The model under review builds one solid part; all positions refer to its coordinate system, in mm. A direction names the side the tool comes from. Round coordinates to 2 decimals unless told otherwise and drop trailing zeros. Write each loop counter-clockwise with the first axis right and the second up, starting at its lowest first coordinate (ties: lowest second). Pieces come first, ordered by that corner, then holes.
Item 1: To check wall thickness, follow L1, parallel to Z at x = 3, y = 260; L2, parallel to Y at x = 27, z = 490; L3, parallel to X at y = 1, z = 622. State the ranges of each line that lie inside material, in increasing order.
Item 2: Draft analysis for pull direction Y (two halves, no side actions). For faces 1 (the face through (4, 270, 0)), 2 (the face through (39, 0, 715)), 3 (the face through (2.465, 155.66, 379.993)), state which applies: +Y half, -Y half, draft (parallel to the pull), parting line (faces both ways), or undercut.
Item 3: Clearance check with flat-ended pins moving along their axes: pin 1 Ø22 at (y, z) = (280, 375) entering from +X; pin 2 Ø5.5 at (x, z) = (1.5, 257.5) entering from -Y; pin 3 Ø9 at (x, z) = (40.09, 640) entering from -Y. State where each tip first meets the part, or that it passes through.
Item 4: Machinability: for faces 4 (the face through (39, 310, 715)), 5 (the face through (5, 157, 715)), which of the approach directions +Z, -Z, +X, -X, +Y, -Y give a long, thin tool a straight path to every point of the face, cutting with its end or side? Answer none if there is none.
Item 5: Add section A-A (z = 1319). Give the boundary of the cut face in (x, y), plus the area to 3 significant figures.
```python
from build123d import *

# Parameters (mm, degrees)
EXTRUDE_1_DEPTH             = 1450
CUT_EXTRUDE_705_DEPTH       = 10
SKETCH_3_R                  = 8.5
CUT_EXTRUDE_1476_DEPTH      = 5
SKETCH_9_R                  = 4
CUT_EXTRUDE_2268_DEPTH      = 10
SKETCH_12_R                 = 6.6
CUT_EXTRUDE_3079_DEPTH      = 10
CUT_EXTRUDE_3564_DEPTH      = 10
SKETCH_17_R                 = 6.6
CUT_EXTRUDE_3911_DEPTH      = 10
FILLET_1_R                  = 10
SKETCH_21_R                 = 4.1
CUT_EXTRUDE_1_DEPTH         = 5
SKETCH_22_R                 = 5.5
CUT_EXTRUDE_4798_DEPTH      = 5
SKETCH_23_R                 = 8.25
CUT_EXTRUDE_5030_DEPTH      = 10
SKETCH_24_R                 = 4.1
CUT_EXTRUDE_2_DEPTH         = 10
HOLE_WIZARD_M61_D           = 6.6
HOLE_WIZARD_M61_DEPTH       = 10
HOLE_WIZARD_M61_CSINK_D     = 13.71
HOLE_WIZARD_M61_CSINK_ANGLE = 90
HOLE_WIZARD_M61_TIP         = 1.982840043


with BuildPart() as part:
    # Эскиз1 → Бобышка-Вытянуть1 (new body)
    with BuildSketch(Plane.XY):
        with BuildLine():
            Line((70, 0), (8, 0))
            ThreePointArc((8, 0), (2.343145751, 2.343145751), (0, 8))
            Line((0, 8), (0, 302))
            ThreePointArc((0, 302), (2.343145751, 307.656854249), (8, 310))
            Line((8, 310), (70, 310))
            Line((70, 310), (70, 305))
            Line((70, 305), (8, 305))
            ThreePointArc((8, 305), (5.878679656, 304.121320344), (5, 302))
            Line((5, 302), (5, 8))
            ThreePointArc((5, 8), (5.878679656, 5.878679656), (8, 5))
            Line((8, 5), (70, 5))
            Line((70, 5), (70, 0))
        make_face()
    extrude(amount=EXTRUDE_1_DEPTH)

    # Эскиз2 → Cut-Extrude 705 (cut)
    with BuildSketch(Plane.ZY):
        with BuildLine():
            Line((350, 125), (0, 125))
            Line((0, 125), (0, 185))
            Line((0, 185), (350, 185))
            ThreePointArc((350, 185), (380, 155), (350, 125))
        make_face()
    extrude(amount=-CUT_EXTRUDE_705_DEPTH, mode=Mode.SUBTRACT)

    # Эскиз3 → Cut-Extrude 1476 (cut, symmetric)
    with BuildSketch(Plane(origin=(5, 0, 0), x_dir=(0, 0, -1), z_dir=(1, 0, 0))):
        with Locations((-225, 280)):
            Circle(SKETCH_3_R)
        with Locations(Location((-225, 30, 0), (0, 0, 180))):
            Circle(SKETCH_3_R)
        with Locations(Location((-375, 280, 0), (0, 0, 180))):
            Circle(SKETCH_3_R)
        with Locations((-375, 30)):
            Circle(SKETCH_3_R)
    extrude(amount=CUT_EXTRUDE_1476_DEPTH, both=True, mode=Mode.SUBTRACT)

    # Эскиз9 → Cut-Extrude 2268 (cut)
    with BuildSketch(Plane.ZY):
        with Locations(Location((740, 260, 0), (0, 0, 270))):
            Circle(SKETCH_9_R)
        with Locations(Location((980, 260, 0), (0, 0, 270))):
            Circle(SKETCH_9_R)
        with BuildLine():
            Line((778, 240), (942, 240))
            ThreePointArc((942, 240), (954.727922061, 245.272077939), (960, 258))
            Line((960, 258), (960, 262))
            ThreePointArc((960, 262), (954.727922061, 274.727922061), (942, 280))
            Line((942, 280), (778, 280))
            ThreePointArc((778, 280), (765.272077939, 274.727922061), (760, 262))
            Line((760, 262), (760, 258))
            ThreePointArc((760, 258), (765.272077939, 245.272077939), (778, 240))
        make_face()
    extrude(amount=-CUT_EXTRUDE_2268_DEPTH, mode=Mode.SUBTRACT)

    # Эскиз12 → Cut-Extrude 3079 (cut)
    with BuildSketch(Plane.ZY):
        with Locations(Location((38, 215, 0), (0, 0, 270))):
            Circle(SKETCH_12_R)
        with Locations(Location((38, 260, 0), (0, 0, 270))):
            Circle(SKETCH_12_R)
        with Locations((38, 95)):
            Circle(SKETCH_12_R)
        with Locations((38, 50)):
            Circle(SKETCH_12_R)
    extrude(amount=-CUT_EXTRUDE_3079_DEPTH, mode=Mode.SUBTRACT)

    # Эскиз13 → Cut-Extrude 3564 (cut)
    with BuildSketch(Plane(origin=(0, 310, 0), x_dir=(1, 0, 0), z_dir=(0, 1, 0))):
        with BuildLine():
            Line((37.5, -166.5), (37.5, -102.5))
            ThreePointArc((37.5, -102.5), (43, -97), (48.5, -102.5))
            Line((48.5, -102.5), (48.5, -166.5))
            ThreePointArc((48.5, -166.5), (43, -172), (37.5, -166.5))
        make_face()
        with BuildLine():
            Line((37.5, -261.5), (37.5, -197.5))
            ThreePointArc((37.5, -197.5), (43, -192), (48.5, -197.5))
            Line((48.5, -197.5), (48.5, -261.5))
            ThreePointArc((48.5, -261.5), (43, -267), (37.5, -261.5))
        make_face()
    extrude(amount=-CUT_EXTRUDE_3564_DEPTH, mode=Mode.SUBTRACT)

    # Эскиз17 → Cut-Extrude 3911 (cut)
    with BuildSketch(Plane(origin=(0, 0, 0), x_dir=(-1, 0, 0), z_dir=(0, -1, 0))):
        with Locations(Location((-36, -562.3, 0), (0, 0, 180))):
            Circle(SKETCH_17_R)
        with Locations(Location((-36, -622.3, 0), (0, 0, 180))):
            Circle(SKETCH_17_R)
    extrude(amount=-CUT_EXTRUDE_3911_DEPTH, mode=Mode.SUBTRACT)

    # Скругление1
    fillet_1_edges = [part.edges().sort_by_distance(p)[0] for p in [
        (2.5, 185, 0),
        (2.5, 125, 0),
    ]]
    fillet(fillet_1_edges, radius=FILLET_1_R)

    # Эскиз21 → Отверстия крепления крышки 1 (cut)
    with BuildSketch(Plane(origin=(0, 310, 0), x_dir=(1, 0, 0), z_dir=(0, 1, 0))):
        with Locations(Location((35, -305.5, 0), (0, 0, 270))):
            Circle(SKETCH_21_R)
    extrude(amount=-CUT_EXTRUDE_1_DEPTH, mode=Mode.SUBTRACT)

    # Эскиз22 → Cut-Extrude 4798 (cut)
    with BuildSketch(Plane.XZ):
        with Locations((40.0885, 500)):
            Circle(SKETCH_22_R)
        with Locations((40.0885, 640)):
            Circle(SKETCH_22_R)
    extrude(amount=-CUT_EXTRUDE_4798_DEPTH, mode=Mode.SUBTRACT)

    # Эскиз23 → Cut-Extrude 5030 (cut)
    with BuildSketch(Plane.XZ):
        with Locations((35, 1347)):
            Circle(SKETCH_23_R)
    extrude(amount=-CUT_EXTRUDE_5030_DEPTH, mode=Mode.SUBTRACT)

    # Эскиз24 → Отверстие крепления крышки 2 (cut)
    with BuildSketch(Plane(origin=(0, 310, 0), x_dir=(1, 0, 0), z_dir=(0, 1, 0))):
        with Locations(Location((35, -1424.5, 0), (0, 0, 270))):
            Circle(SKETCH_24_R)
    extrude(amount=-CUT_EXTRUDE_2_DEPTH, mode=Mode.SUBTRACT)

    # Зенковка для винта с потайной головкой и внутренним шестигранником M61
    with Locations(Plane.XZ):
        with Locations((40, 1432)):
            CounterSinkHole(HOLE_WIZARD_M61_D / 2, HOLE_WIZARD_M61_CSINK_D / 2, depth=HOLE_WIZARD_M61_DEPTH, counter_sink_angle=HOLE_WIZARD_M61_CSINK_ANGLE)
            with Locations((0, 0, -(HOLE_WIZARD_M61_DEPTH + HOLE_WIZARD_M61_TIP / 2))):  # 118° drill point
                Cone(0, HOLE_WIZARD_M61_D / 2, HOLE_WIZARD_M61_TIP, mode=Mode.SUBTRACT)


solid = part.part
```
Numbers:
1. L1: z = 0 to 31.4, 44.6 to 736, 744 to 760, 960 to 976, 984 to 1450
1. L2: y = 0 to 5, 305 to 310
1. L3: x = 4.13 to 29.41, 42.59 to 70
2. face 1: draft
2. face 2: -Y half
2. face 3: undercut
3. pin 1: stops at x = 5
3. pin 2: stops at y = 0.93
3. pin 3: stops at y = 305
4. face 4: +Z, -Z, +X, -X, +Y
4. face 5: +Z, -Z, +X
5. outline: (0, 8) arc R8 ccw to (8, 0) - (70, 0) - (70, 5) - (8, 5) arc R3 cw to (5, 8) - (5, 302) arc R3 cw to (8, 305) - (70, 305) - (70, 310) - (8, 310) arc R8 ccw to (0, 302) - close
5. area: 2,180 mm2
